Part print with two shaded views. Sizes in mm from the minimum x, y, z corner. A direction names the side the tool comes from. Give positions to 0.01 mm unless a question says otherwise; leave off trailing zeros. Write each loop counter-clockwise with the first axis right and the second up, starting at its lowest first coordinate (ties: lowest second). Pieces come first, ordered by that corner, then holes. Notation, with made-up numbers: M 69,6 L 81,6 A18 cw 81,24 Z; hole C 49,88 d3. An arc over 180 degrees is marked long. Return JSON: item names as keys, results as strings. Group by question number.
Q1. Band-saw the part on A-A, the plane y = 18. Give the cut face in (x, z) (1 decimal).
Q2. Band-saw the part on B-B, the plane y = 3. Give the cut face in (x, z) (1 decimal).
Q3. Wall check: probe 1 along X at (y, z) = (12.5, 5) (1 decimal); probe 2 along Y at (x, z) = (2.5, 5.75); probe 3 along Z at (x, y) = (5, 28). Give the ranges that are in metal, low to high.
Q4. Flat gauge pins, fed straight in: pin 1 Ø2 at (x, y) = (8, 19) entering from +Z (1 decimal); pin 2 Ø1 at (x, z) = (1, 7) entering from -Y (1 decimal); pin 3 Ø3 at (x, y) = (4, 32.5) entering from +Z; pin 4 Ø1 at (y, z) = (31, 8) entering from -X. Where does each tip first touch, or does it go through?
Q5. Tool access for the marked faces 1 and 2: list every direction of +Z, -Z, +X, -X, +Y, -Y with a clear straight run to the whole face (end or side of a thin tool).
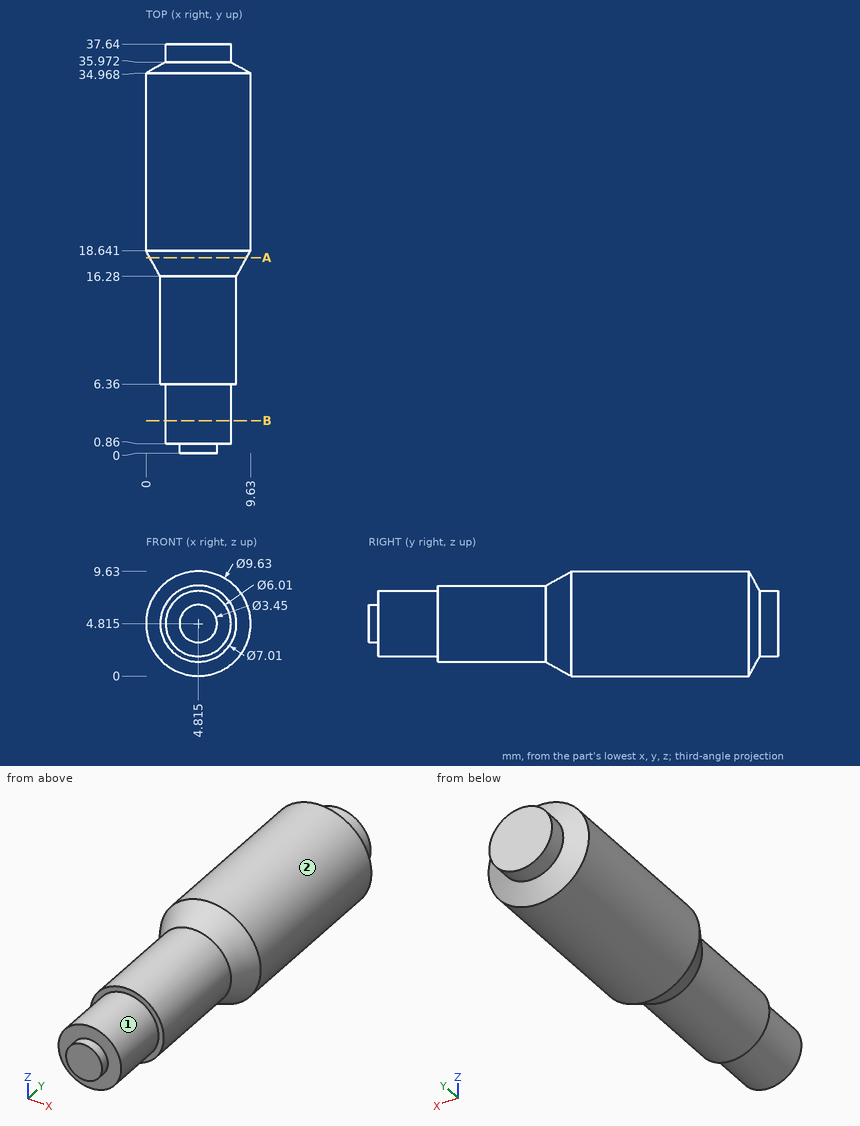
From the geometry:
{
 "1": {"outline": "C 4.8,4.8 d8.9"},
 "2": {"outline": "C 4.8,4.8 d6"},
 "3": {"probe 1": "x = 1.3 to 8.3", "probe 2": "y = 0.86 to 37.64", "probe 3": "z = 0 to 9.63"},
 "4": {"pin 1": "stops at z = 9.1", "pin 2": "stops at y = 17", "pin 3": "stops at z = 9.63", "pin 4": "stops at x = 0.82"},
 "5": {"face 1": "-Y", "face 2": "+Y, -Y"}
}
